Autodesk Inventor part; units mm, degrees
ref_plane "Start Plane" through (0, 0, -7.968) normal (0, 0, 1) x (1, 0, 0)
ref_plane "End Plane" through (0, 0, 352.4706) normal (0, 0, 1) x (1, 0, 0)
ref_plane "Work Plane4" through (-10, 0, -7.968) normal (0.3492, 0, -0.9371) x (-0.9371, 0, -0.3492)
ref_plane "Start Plane" through (0, 0, -7.968) normal (0, 0, 1) x (1, 0, 0)
ref_plane "End Plane" through (0, 0, 352.4706) normal (0, 0, 1) x (1, 0, 0)
sketch "Sketch" plane through (0, 0, 0) normal (0, 0, 1) x (1, 0, 0)
  line L0 (-10, -7) -> (-10, 7)
  line L1 (-7, 10) -> (7, 10)
  line L2 (10, 7) -> (10, -7)
  line L3 (7, -10) -> (-7, -10)
  arc A0 (-10, -7) -> (-7, -10) centre (-7, -7) ccw
  arc A1 (-7, 10) -> (-10, 7) centre (-7, 7) ccw
  arc A2 (10, 7) -> (7, 10) centre (7, 7) ccw
  arc A3 (7, -10) -> (10, -7) centre (7, -7) ccw
  arc A4 (-7, 8) -> (-8, 7) centre (-7, 7) ccw
  line L4 (-7, 8) -> (7, 8)
  arc A5 (8, 7) -> (7, 8) centre (7, 7) ccw
  line L5 (8, 7) -> (8, -7)
  arc A6 (7, -8) -> (8, -7) centre (7, -7) ccw
  line L6 (7, -8) -> (-7, -8)
  arc A7 (-8, -7) -> (-7, -8) centre (-7, -7) ccw
  line L7 (-8, -7) -> (-8, 7)
  line L8 (0, 14.8698) -> (0, -14.8698) construction
  line L9 (-14.8698, 0) -> (14.8698, 0) construction
  dimension "d7" = 3
  dimension "d10" = 20
  dimension "d11" = 20
  dimension "d12" = 2
  dimension "d15" = 10
  dimension "d16" = 10
extrude "Body" add sketch "Sketch" along normal up to surface (360.4385 mm away) from surface at -7.968
sketch "Sketch3" plane through (0, 0, 0) normal (0, 0, 1) x (1, 0, 0)
  line L0 (0, 0) -> (10, 0)
ref_plane "Work Plane3" through (0, 0, 0) normal (0, -1, 0) x (1, 0, 0)
sketch "Sketch4" plane through (0, 0, 0) normal (0, -1, 0) x (1, 0, 0)
  line L0 (-2, -7.968) -> (12, -7.968)
  line L1 (-2, 352.4706) -> (12, 352.4706)
  dimension "d18" = 360.4385
ref_plane "Work Plane4" through (-10, 0, -7.968) normal (0.3492, 0, -0.9371) x (-0.9371, 0, -0.3492)
split "Split1" plane through (-10, 0, -7.968) removes the side toward (0.3492, 0, -0.9371)
ref_plane "Work Plane5" through (0, -10, 352.4706) normal (0, 0.7897, 0.6134) x (1, 0, 0)
split "Split2" plane through (0, -10, 352.4706) removes the side toward (0, 0.7897, 0.6134)
ref_plane "Work Plane6" through (12.1423, 0, 340.8474) normal (0.7562, 0, 0.6544) x (0.6544, 0, -0.7562)
split "Split3" plane through (12.1423, 0, 340.8474) removes the side toward (0.7562, 0, 0.6544)
ref_plane "Work Plane7" through (-1.2506, 0, 351.7391) normal (-0.6544, 0, 0.7562) x (0.7562, 0, 0.6544)
split "Split4" plane through (-1.2506, 0, 351.7391) removes the side toward (-0.6544, 0, 0.7562)
equation "\"d7\" = G_IR"
equation "\"d10\" = G_H"
equation "\"d11\" = G_W"
equation "\"d12\" = G_T"
equation "\"d15\" = 0.5 * d10"
equation "\"d16\" = 0.5 * d11"
equation "\"d3\" = G_L"
equation "\"G_W\" = 20"
equation "\"G_H\" = 20"
equation "\"G_T\" = 2"
equation "\"G_IR\" = 3"
equation "\"G_L\" = d18"
equation "\"G_OFFSET_START\" = 7.96796"
equation "\"G_OFFSET_END\" = 12.87375"
equation "\"d13\" = -G_OFFSET_START"
equation "\"d14\" = G_OFFSET_END + B_L"
equation "\"B_L\" = 339.59682"
properties part number "ISO 12633-2 - 20x20x2 - 360,44  sideplan 1 bagerste stolpe" material "Steel, Mild"
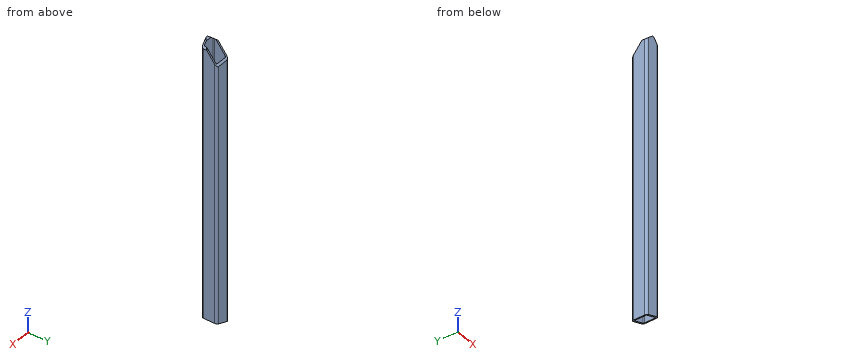
The model under review builds one solid part; all positions refer to its coordinate system, in mm. Coordinates: 2 decimals unless noted, no trailing zeros. Loops run counter-clockwise (first coordinate to the right, second up) from the corner with the lowest first, then second, coordinate; pieces in that order, holes last. Notation, with made-up numbers: (86.5, 70) -> (137.5, 70) arc R5 ccw to (137.5, 74) -> close; hole circle Ø5 at (-4.75, 89.5). An arc over 180 degrees is marked (long way). Use a Markdown table: item, result. Add a question column.
1. Clearance check with a flat-ended pin moving along its axis: pin 1 Ø2 at (x, z) = (7.5, 36) entering from -Y. State where the tip first meets the part, or that it passes through.
2. Add section A-A on z = 23. Write out the cut boundary in (x, y), plus the area to 3 significant figures.
3. To check wall thickness, follow line 1 (X direction, y = 3.5, z = 287.5); line 2 (Z direction, x = 8.75, y = 3). State the ranges of each line that lie inside material, in increasing order.
4. Add section B-B on y = 0.5. Write out the cut boundary in (x, z).
Returned:
| question | item | result |
|---|---|---|
| 1 | pin 1 | stops at y = -10 |
| 2 | outline | (-10, -7) arc R3 ccw to (-7, -10) -> (7, -10) arc R3 ccw to (10, -7) -> (10, 7) arc R3 ccw to (7, 10) -> (-7, 10) arc R3 ccw to (-10, 7) -> close; hole (-8, -7) arc R1 ccw to (-7, -8) -> (7, -8) arc R1 ccw to (8, -7) -> (8, 7) arc R1 ccw to (7, 8) -> (-7, 8) arc R1 ccw to (-8, 7) -> close |
| 2 | area | 137 mm² |
| 3 | line 1 | x = -10 to -8, 8 to 10 |
| 3 | line 2 | z = -0.98 to 335.73 |
| 4 | outline | (-10, -7.97) -> (-8, -7.22) -> (-8, 338.95) -> (-10, 338.95) -> close; (8, -1.26) -> (10, -0.52) -> (10, 338.95) -> (8, 338.95) -> close |
